Check sheet for the modelled part. Datum: model origin and axes. Units: mm. A direction names the side the tool comes from. Give positions to 0.01 mm unless a question says otherwise; leave off trailing zeros. Order: outer loops, then holes, each group sorted by start corner. A loop starts at its lowest first (then second) coordinate and runs counter-clockwise, first axis right, second up.
```python
from build123d import *

# Parameters (mm, degrees)
SKETCH1_W           = 150
SKETCH1_H           = 150
BOSS_EXTRUDE1_DEPTH = 10
SKETCH2_W           = 50
SKETCH2_H           = 60
BOSS_EXTRUDE2_DEPTH = 40
BOSS_EXTRUDE3_DEPTH = 60
SKETCH4_R           = 10
CUT_EXTRUDE1_DEPTH  = 60
SKETCH5_W           = 30
SKETCH5_H           = 30
CUT_EXTRUDE2_DEPTH  = 50
SKETCH6_R           = 25
CUT_EXTRUDE3_DEPTH  = 30


with BuildPart() as part:
    # Sketch1 → Boss-Extrude1 (new body)
    with BuildSketch(Plane(origin=(0, 0, 0), x_dir=(1, 0, 0), z_dir=(0, 1, 0))):
        Rectangle(SKETCH1_W, SKETCH1_H)
    extrude(amount=BOSS_EXTRUDE1_DEPTH)

    # Sketch2 → Boss-Extrude2 (add)
    with BuildSketch(Plane(origin=(0, 10, 0), x_dir=(1, 0, 0), z_dir=(0, 1, 0))):
        Rectangle(SKETCH2_W, SKETCH2_H)
    extrude(amount=BOSS_EXTRUDE2_DEPTH)

    # Sketch3 → Boss-Extrude3 (add)
    with BuildSketch(Plane.XY.offset(30)):
        with BuildLine():
            Line((-25, 50), (25, 50))
            ThreePointArc((25, 50), (0, 75), (-25, 50))
        make_face()
    extrude(amount=-BOSS_EXTRUDE3_DEPTH)

    # Sketch4 → Cut-Extrude1 (cut)
    with BuildSketch(Plane.XY.offset(30)):
        with Locations((0, 50)):
            Circle(SKETCH4_R)
    extrude(amount=-CUT_EXTRUDE1_DEPTH, mode=Mode.SUBTRACT)

    # Sketch5 → Cut-Extrude2 (cut)
    with BuildSketch(Plane.ZY.offset(25)):
        with Locations((0, 60)):
            Rectangle(SKETCH5_W, SKETCH5_H)
    extrude(amount=-CUT_EXTRUDE2_DEPTH, mode=Mode.SUBTRACT)

    # Sketch6 → Cut-Extrude3 (cut)
    with BuildSketch(Plane.XY.offset(-15)):
        with Locations((0, 50)):
            Circle(SKETCH6_R)
    extrude(amount=CUT_EXTRUDE3_DEPTH, mode=Mode.SUBTRACT)


solid = part.part
```
(1) Set-up check for faces 5 (the face through (0, 36, 30)), 6 (the face through (0, 25, 0)), 7 (the face through (-25, 30, 0)), 8 (the face through (0, 36, -30)): record each of +Z, -Z, +X, -X, +Y, -Y from which the full face is reachable in a straight line by a thin tool's end or side.
Response values:
face 5: +Z, +X, -X, +Y
face 6: +Y
face 7: +Z, -Z, -X, +Y
face 8: -Z, +X, -X, +Y
(2) Material ranges on L1, parallel to X at y = 50, z = -26; L2, parallel to Z at x = -11.5, y = 46; L3, parallel to Y at x = 0, z = -26.75, recorded low to high.
Response values:
L1: x = -25 to -10, 10 to 25
L2: z = -30 to -15, 15 to 30
L3: y = 0 to 40, 60 to 75
(3) Cross-section at B-B on y = 52.5. Enter the section's corners in (x, z), then the cut area to 3 significant figures.
Response values:
outline: (-24.87, -30) - (-9.68, -30) - (-9.68, -15) - (-24.87, -15) - close; (-24.87, 15) - (-9.68, 15) - (-9.68, 30) - (-24.87, 30) - close; (9.68, -30) - (24.87, -30) - (24.87, -15) - (9.68, -15) - close; (9.68, 15) - (24.87, 15) - (24.87, 30) - (9.68, 30) - close
area: 912 mm2
(4) Gauge pin test, flat ends, axial feed: pin 1 Ø15 at (x, y) = (-11.5, 57.5) entering from -Z; pin 2 Ø4 at (x, z) = (-30, -19) entering from +Y; pin 3 Ø12 at (y, z) = (30, -11.5) entering from -X. Record the tip position at first contact, or that the pin passes through.
Response values:
pin 1: stops at z = -30
pin 2: stops at y = 10
pin 3: stops at x = -25
(5) Release check for a two-part mould opening along Y. For faces 1 (the face through (25, 30, 0)), 2 (the face through (-2.17, 40.24, 22.6)), 3 (the face through (-2.17, 40.24, -22.39)), 4 (the face through (-1, 0, -1)) record: released by +Y, released by -Y, zero draft, split by the parting line, or undercut.
Response values:
face 1: zero draft
face 2: undercut
face 3: undercut
face 4: released by -Y
(6) Cross-section at A-A on x = 0. Enter the section's corners in (y, z).
Response values:
outline: (0, -75) - (10, -75) - (10, -30) - (40, -30) - (40, -15) - (25, -15) - (25, 15) - (40, 15) - (40, 30) - (10, 30) - (10, 75) - (0, 75) - close; (60, -30) - (75, -30) - (75, -15) - (60, -15) - close; (60, 15) - (75, 15) - (75, 30) - (60, 30) - close
(7) Cross-section at C-C on z = 3.5. Enter the section's corners in (x, y).
Response values:
outline: (-75, 0) - (75, 0) - (75, 10) - (25, 10) - (25, 45) - (24.49, 45) arc R25 cw to (-24.49, 45) - (-25, 45) - (-25, 10) - (-75, 10) - close
(8) Cross-section at D-D on x = -16. Enter the section's corners in (y, z), then the cut area to 3 significant figures.
Response values:
outline: (0, -75) - (10, -75) - (10, -30) - (69.21, -30) - (69.21, -15) - (30.79, -15) - (30.79, 15) - (69.21, 15) - (69.21, 30) - (10, 30) - (10, 75) - (0, 75) - close
area: 3,900 mm2
